Verification items for the finished model (mm, model axes). A direction names the side the tool comes from. Give positions to 0.01 mm unless a question says otherwise; leave off trailing zeros. Order: outer loops, then holes, each group sorted by start corner. A loop starts at its lowest first (then second) coordinate and runs counter-clockwise, first axis right, second up.
(1) Access from +Z, -Z, +X, -X, +Y, -Y to the whole of each face (thin tool, end or side, straight path). Record for faces 5 (the face through (-10, 11.85, 1)), 6 (the face through (11.45, 10, 6)), 7 (the face through (-12.7, 8.35, 6)).
(2) Sectioned sample at D-D on x = 4.5. Record the cut outline in (y, z).
(3) Scan lines: L1, parallel to Z at x = 14.45, y = 7.65; L2, parallel to Y at x = 3.5, z = 5; L3, parallel to X at y = 0, z = 5.5. Record each from-to range of solid material in increasing order.
(4) Sectioned sample at B-B on z = 9.25. Record the cut outline in (x, y), plus the area to 3 significant figures.
(5) Mould release check, pull along Z, two halves, no side actions. Record for faces 1 (the face through (-10, 11.85, 11)), 2 (the face through (2.8, 13.6, 6.1)), 3 (the face through (-12.95, 7.17, 6.15)), 4 (the face through (0, 0, 0)): pulls with the +Z half, pulls with the -Z half, needs draft (parallel to the pull), parting line crosses it, or undercut.
(6) Gauge pin test, flat ends, axial feed: pin 1 (1.3 mm diameter, centred on x = -13.5, z = 5.5, fed in from +Y); pin 2 (2.5 mm diameter, centred on x = 14.45, z = 6.1, fed in from +Y); pin 3 (5 mm diameter, centred on x = -14.45, z = 6.1, fed in from -Y); pin 4 (5 mm diameter, centred on x = -8.5, z = 1.5, fed in from +Y). Record the tip position at first contact, or that the pin passes through.
(7) Sectioned sample at C-C on y = -9. Record the cut outline in (x, z), plus the area to 3 significant figures.
(8) Sectioned sample at A-A on x = -14.45. Record the cut outline in (y, z).
```python
from build123d import *

# Parameters (mm, degrees)
CROQUIS1_W              = 22.9
CROQUIS1_H              = 23.7
CROQUIS1_W_2            = 4.5
CROQUIS1_H_2            = 2.4
SALIENTE_EXTRUIR1_DEPTH = 12.2
CROQUIS2_R              = 6.1
CROQUIS2_R_2            = 2.05
SALIENTE_EXTRUIR2_DEPTH = 3.5
SALIENTE_EXTRUIR3_START = 3.5
CROQUIS2_3_R            = 2.05
SALIENTE_EXTRUIR3_DEPTH = 2
CORTAR_EXTRUIR2_REACH   = 30.483
CROQUIS3_R              = 1.5


with BuildPart() as part:
    # Croquis1 → Saliente-Extruir1 (new body)
    with BuildSketch(Plane.XY):
        Rectangle(CROQUIS1_W, CROQUIS1_H)
        with Locations((-13.7, 7.15)):
            Rectangle(CROQUIS1_W_2, CROQUIS1_H_2)
        with Locations((13.7, 7.15)):
            Rectangle(CROQUIS1_W_2, CROQUIS1_H_2)
    extrude(amount=SALIENTE_EXTRUIR1_DEPTH)

    # Croquis2 → Saliente-Extruir2 (add)
    # profile 1 of 3: a face of its own
    with BuildSketch(Plane(origin=(0, 11.85, 0), x_dir=(1, 0, 0), z_dir=(0, 1, 0))):
        with BuildLine():
            ThreePointArc((0.405532787, -4.079148115), (0.663266583, -5.075), (0.75, -6.1))
            ThreePointArc((0.75, -6.1), (0.663266583, -7.125), (0.405532787, -8.120851885))
            ThreePointArc((0.405532787, -8.120851885), (2.8, -6.1), (0.405532787, -4.079148115))
        make_face()
    # profile 2 of 3: a face of its own
    with BuildSketch(Plane(origin=(0, 11.85, 0), x_dir=(1, 0, 0), z_dir=(0, 1, 0))):
        with Locations((-5.35, -6.1)):
            Circle(CROQUIS2_R)
        with Locations((-5.35, -6.1)):
            Circle(CROQUIS2_R_2, mode=Mode.SUBTRACT)
    # profile 3 of 3: a face of its own
    with BuildSketch(Plane(origin=(0, 11.85, 0), x_dir=(1, 0, 0), z_dir=(0, 1, 0))):
        with Locations((-5.35, -6.1)):
            Circle(CROQUIS2_R_2)
    extrude(amount=SALIENTE_EXTRUIR2_DEPTH)

    # Croquis2<3> → Saliente-Extruir3 (add)
    with BuildSketch(Plane(origin=(0, 11.85, 0), x_dir=(1, 0, 0), z_dir=(0, 1, 0)).offset(SALIENTE_EXTRUIR3_START)):
        with Locations(Location((-5.35, -6.1, 0), (0, 0, 270))):
            Circle(CROQUIS2_3_R)
    extrude(amount=SALIENTE_EXTRUIR3_DEPTH)

    # Croquis3 → Cortar-Extruir2 (cut, up to next)
    with BuildSketch(Plane(origin=(0, 8.35, 0), x_dir=(1, 0, 0), z_dir=(0, 1, 0)), mode=Mode.PRIVATE) as cortar_extruir2_sk1:
        with Locations((-14.45, -6.1)):
            Circle(CROQUIS3_R)
    cortar_extruir2_tool1 = extrude(cortar_extruir2_sk1.sketch, amount=-CORTAR_EXTRUIR2_REACH, mode=Mode.PRIVATE) & part.part
    # Croquis3 → Cortar-Extruir2 (cut, up to next)
    with BuildSketch(Plane(origin=(0, 8.35, 0), x_dir=(1, 0, 0), z_dir=(0, 1, 0)), mode=Mode.PRIVATE) as cortar_extruir2_sk2:
        with BuildLine():
            ThreePointArc((-15.469803903, -7.2), (-15.824719218, -6.700122548), (-15.95, -6.1))
            Line((-15.95, -6.1), (-15.95, -7.2))
            Line((-15.95, -7.2), (-15.469803903, -7.2))
        make_face()
    cortar_extruir2_tool2 = extrude(cortar_extruir2_sk2.sketch, amount=-CORTAR_EXTRUIR2_REACH, mode=Mode.PRIVATE) & part.part
    # Croquis3 → Cortar-Extruir2 (cut, up to next)
    with BuildSketch(Plane(origin=(0, 8.35, 0), x_dir=(1, 0, 0), z_dir=(0, 1, 0)), mode=Mode.PRIVATE) as cortar_extruir2_sk3:
        with BuildLine():
            Line((-15.469803903, -5), (-15.95, -5))
            Line((-15.95, -5), (-15.95, -6.1))
            ThreePointArc((-15.95, -6.1), (-15.824719218, -5.499877452), (-15.469803903, -5))
        make_face()
    cortar_extruir2_tool3 = extrude(cortar_extruir2_sk3.sketch, amount=-CORTAR_EXTRUIR2_REACH, mode=Mode.PRIVATE) & part.part
    cortar_extruir2_1 = cortar_extruir2_tool1.solids().sort_by_distance((-14.45, 8.35, 6.1))[0]
    add(cortar_extruir2_1, mode=Mode.SUBTRACT)
    cortar_extruir2_2 = cortar_extruir2_tool2.solids().sort_by_distance((-15.810988, 8.35, 6.934581))[0]
    add(cortar_extruir2_2, mode=Mode.SUBTRACT)
    cortar_extruir2_3 = cortar_extruir2_tool3.solids().sort_by_distance((-15.810988, 8.35, 5.265419))[0]
    add(cortar_extruir2_3, mode=Mode.SUBTRACT)
    cortar_extruir2 = cortar_extruir2_1 + cortar_extruir2_2 + cortar_extruir2_3  # Cortar-Extruir2 as one shape, for the pattern or mirror that repeats it

    # Simetría1: Cortar-Extruir2 across plane
    add(cortar_extruir2.mirror(Plane(origin=(0, 0, 0), x_dir=(0, 0, 1), z_dir=(1, 0, 0))), mode=Mode.SUBTRACT)


solid = part.part
```
Ans:
1. face 5: -Z, -X, +Y
1. face 6: +Z, -Z, +X, +Y
1. face 7: +Z, -Z, -X, +Y
2. outline: (-11.85, 0) - (11.85, 0) - (11.85, 12.2) - (-11.85, 12.2) - close
3. L1: z = 0 to 4.6, 7.6 to 12.2
3. L2: y = -11.85 to 11.85
3. L3: x = -11.45 to 11.45
4. outline: (-15.95, 5.95) - (-11.45, 5.95) - (-11.45, -11.85) - (11.45, -11.85) - (11.45, 5.95) - (15.95, 5.95) - (15.95, 8.35) - (11.45, 8.35) - (11.45, 11.85) - (-0.13, 11.85) - (-0.13, 15.35) - (-10.57, 15.35) - (-10.57, 11.85) - (-11.45, 11.85) - (-11.45, 8.35) - (-15.95, 8.35) - close
4. area: 601 mm2
5. face 1: needs draft
5. face 2: parting line crosses it
5. face 3: undercut
5. face 4: pulls with the -Z half
6. pin 1: stops at y = 8.35
6. pin 2: passes through
6. pin 3: stops at y = 5.95
6. pin 4: stops at y = 15.35
7. outline: (-11.45, 0) - (11.45, 0) - (11.45, 12.2) - (-11.45, 12.2) - close
7. area: 279 mm2
8. outline: (5.95, 0) - (8.35, 0) - (8.35, 4.6) - (5.95, 4.6) - close; (5.95, 7.6) - (8.35, 7.6) - (8.35, 12.2) - (5.95, 12.2) - close
